Here's how the part is built. I have some questions about the finished solid (model axes, mm). A direction names the side the tool comes from. Coordinates: 2 decimals unless noted, no trailing zeros. Loops run counter-clockwise (first coordinate to the right, second up) from the corner with the lowest first, then second, coordinate; pieces in that order, holes last. Notation, with made-up numbers: M -4.5,54.25 L 19.5,54.25 A31 ccw 19.5,84.25 Z; hole C 33.5,8 d8. An arc over 180 degrees is marked long. Use one line per item in the form item = value. Start each with the question number.
(1) Thinking about a two-plate mould opening in X: for faces 6 (the flat face through (0, 25.073, -7)), 7 (the flat face through (44.208, 19.436, -5.93)), which applies, +X half, -X half, draft (parallel to the pull), parting line (faces both ways), or undercut?
(2) Imagine slicing it at B-B, the plane x = 23. Please give me the cut outline in (y, z).
(3) Will these pins go through, and if not, where does the flat tip stop? P1, Ø1.3, axis at x = 38, y = -24, coming from the +Z side; P2, Ø2.5, axis at x = 46.75, y = -21.82, coming from the +Z side; P3, Ø1.3, axis at y = -24.5, z = -2.5, coming from the -X side; P4, Ø1.3, axis at y = -24, z = -3.5, coming from the -X side.
(4) Imagine slicing it at A-A, the plane y = 9. Please give me the cut outline in (x, z), and give its area (3 significant figures).
(5) Imagine slicing it at C-C, the plane x = 39. Please give me the cut outline in (y, z), and give its area (3 significant figures).
(6) Please list where these lines run through material, in increasing order: L1, parallel to X at y = 13.5, z = -7; L2, parallel to Y at x = 25, z = -2; L3, parallel to X at y = -18.5, z = -10.
(7) On a 3-axis mill with a long thin cutter (end or side, diameter ignored), from which of +Z, -Z, +X, -X, +Y, -Y can I reach the whole of each face in a straight line? I mean faces 1 (the cylindrical face through (35.76, 4.08, -12.01)), 2 (the cylindrical face through (41.187, 24.178, -6.158)), 3 (the flat face through (42.965, -20, -6)), 4 (the flat face through (-1, -24.85, -7)), 5 (the flat face through (0, 24, -1.865)). Say none if no direction works.
```python
from build123d import *

# Parameters (mm, degrees)
SKETCH008_R     = 1.539175
SKETCH008_R_2   = 1.523329
SKETCH008_R_3   = 1.533201
SKETCH008_R_4   = 1.490189
PAD006_DEPTH    = 12
POCKET002_DEPTH = 10
SKETCH010_W     = 12.5
SKETCH010_H     = 5.5
SKETCH010_W_2   = 7
SKETCH010_H_2   = 3.5
SKETCH010_H_3   = 1.2
SKETCH010_W_3   = 8.5
SKETCH010_H_4   = 3
SKETCH010_W_4   = 15
SKETCH010_H_5   = 2.5
POCKET003_DEPTH = 5
SKETCH011_R     = 2.5
SKETCH011_W     = 18.47
SKETCH011_H     = 1
POCKET004_DEPTH = 5
SKETCH012_R     = 1
POCKET005_DEPTH = 5


with BuildPart() as part:
    # Sketch008 → Pad006 (new body)
    with BuildSketch(Plane.XY):
        with BuildLine():
            add(Edge.make_bspline(
                [(49.8242, 22.201212), (49.508362, 24.731634), (47.160099, 25.0727)],
                knots=[0, 0, 0, 1, 1, 1], degree=2))
            Line((47.160099, 25.0727), (-47.5558, 25.0727))
            add(Edge.make_bspline(
                [(-47.5558, 25.0727), (-49.764992, 24.657032), (-50.191277, 22.540522)],
                knots=[0, 0, 0, 1, 1, 1], degree=2))
            Line((-50.191277, 22.540522), (-50.191277, -22.264349))
            add(Edge.make_bspline(
                [(-50.191277, -22.264349), (-49.80262, -24.340702), (-47.5557, -24.8503)],
                knots=[0, 0, 0, 1, 1, 1], degree=2))
            Line((-47.5557, -24.8503), (47.181141, -24.8503))
            add(Edge.make_bspline(
                [(47.181141, -24.8503), (49.487186, -24.462395), (49.8242, -22.0108)],
                knots=[0, 0, 0, 1, 1, 1], degree=2))
            Line((49.8242, -22.0108), (49.8242, 22.201212))
        make_face()
        with Locations((-47.115311, 21.916405)):
            Circle(SKETCH008_R, mode=Mode.SUBTRACT)
        with Locations((46.738178, 21.927752)):
            Circle(SKETCH008_R_2, mode=Mode.SUBTRACT)
        with Locations((-47.112675, -21.823126)):
            Circle(SKETCH008_R_3, mode=Mode.SUBTRACT)
        with Locations((46.75103, -21.816845)):
            Circle(SKETCH008_R_4, mode=Mode.SUBTRACT)
    extrude(amount=PAD006_DEPTH)

    # Sketch009 (on Face14 of Pad006) → Pocket002 (cut)
    with BuildSketch(Plane.XY.offset(12)):
        Polygon((-44.059395, 23.3085), (-44.059395, 19.16888), (-47.975544, 17.274294), (-47.975544, -18.868563), (-43.311943, -18.868563), (-43.311943, -23.240685), (42.964558, -23.240685), (42.964558, -16.391027), (48.211094, -16.391027), (48.211094, 17.711506), (44.567665, 17.711506), (43.838982, 21.209202), (43.838982, 23.3085), align=None)
    extrude(amount=-POCKET002_DEPTH, mode=Mode.SUBTRACT)

    # Sketch010 (on Face10 of Pocket002) → Pocket003 (cut)
    with BuildSketch(Plane.XZ.offset(24.8503)):
        with Locations((35.071653, 9.29913)):
            Rectangle(SKETCH010_W, SKETCH010_H)
        with Locations((15.86862, 10.28645)):
            Rectangle(SKETCH010_W_2, SKETCH010_H_2)
        with Locations((-1.705669, 11.417012)):
            Rectangle(SKETCH010_W_2, SKETCH010_H_3)
        with Locations((-16.516187, 10.547991)):
            Rectangle(SKETCH010_W_3, SKETCH010_H_4)
        with Locations((-33.384749, 10.757572)):
            Rectangle(SKETCH010_W_4, SKETCH010_H_5)
    extrude(amount=-POCKET003_DEPTH, mode=Mode.SUBTRACT)

    # Sketch011 (on Face23 of Pocket003) → Pocket004 (cut)
    with BuildSketch(Plane.XZ.offset(-23.3085)):
        with Locations((-38.509063, 7.8)):
            Circle(SKETCH011_R)
        with Locations((38.877759, 7.8)):
            Circle(SKETCH011_R)
        with Locations((0.011538, 11.635367)):
            Rectangle(SKETCH011_W, SKETCH011_H)
    extrude(amount=-POCKET004_DEPTH, mode=Mode.SUBTRACT)

    # Sketch012 (on Face4 of Pocket004) → Pocket005 (cut)
    with BuildSketch(Plane(origin=(0, 0, 0), x_dir=(1, 0, 0), z_dir=(0, 0, -1))):
        with Locations((34.805111, -4.37996)):
            Circle(SKETCH012_R)
        with Locations((36.121971, 0.316835)):
            Circle(SKETCH012_R)
        with Locations((30.722851, 0.316835)):
            Circle(SKETCH012_R)
        with Locations((36.165867, -2.272987)):
            Circle(SKETCH012_R)
        with Locations((33.400463, -2.185196)):
            Circle(SKETCH012_R)
        with Locations((35.02459, 2.622291)):
            Circle(SKETCH012_R)
        with Locations((31.995813, 2.578395)):
            Circle(SKETCH012_R)
        with Locations((32.039707, -4.400955)):
            Circle(SKETCH012_R)
        with Locations((30.766747, -2.185196)):
            Circle(SKETCH012_R)
        with Locations((33.400463, 0.36073)):
            Circle(SKETCH012_R)
    extrude(amount=-POCKET005_DEPTH, mode=Mode.SUBTRACT)


with BuildPart() as part_1:
    # Body003 placement: moved
    add(part.part.moved(Location((0, 0, -13))))


solid = part_1.part
```
Answer:
q1.face_6 = draft
q1.face_7 = undercut
q2.outline = M -24.85,-13 L 25.07,-13 L 25.07,-1 L 23.31,-1 L 23.31,-11 L -23.24,-11 L -23.24,-1 L -24.85,-1 Z
q3.P1 = -6.45
q3.P2 = through
q3.P3 = -49.43
q3.P4 = -49.8
q4.outline = M -50.19,-13 L 49.82,-13 L 49.82,-1 L 48.21,-1 L 48.21,-11 L -47.98,-11 L -47.98,-1 L -50.19,-1 Z
q4.area = 238 mm²
q5.outline = M -24.85,-13 L 25.07,-13 L 25.07,-7.7 L 23.31,-7.7 L 23.31,-11 L -23.24,-11 L -23.24,-6.45 L -24.85,-6.45 Z; M 23.31,-2.7 L 25.07,-2.7 L 25.07,-1 L 23.31,-1 Z
q5.area = 116 mm²
q6.L1 = -50.19 to -47.98, 48.21 to 49.82
q6.L2 = -24.85 to -23.24, 23.31 to 25.07
q6.L3 = -50.19 to -47.98, 42.96 to 49.82
q7.face_1 = +Z, -Z
q7.face_2 = +Y
q7.face_3 = +Z
q7.face_4 = +Z, -Z, +X, -X, -Y
q7.face_5 = +Z, +Y
